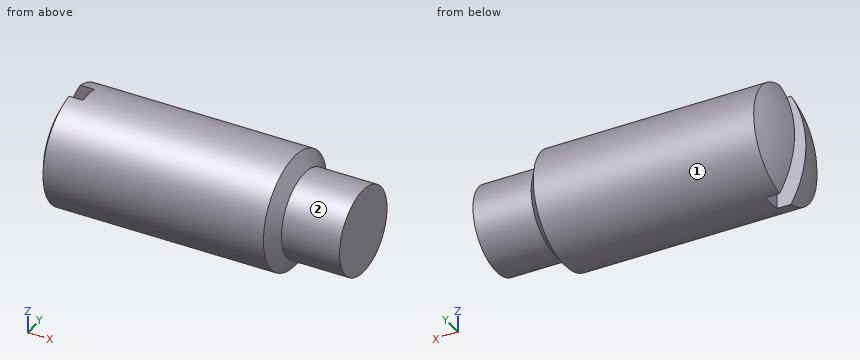
from build123d import *

# Parameters (mm, degrees)
SKETCH2_W  = 19.05
SKETCH2_H  = 3.4036
SLOT_DEPTH = 4.9022


with BuildPart() as part:
    # BodySke → BaseBody (revolve)
    with BuildSketch(Plane.XY, mode=Mode.PRIVATE) as basebody_sk:
        with BuildLine():
            Line((41.0718, 7.1374), (50.8, 7.1374))
            Line((50.8, 7.1374), (50.8, 0))
            Line((50.8, 0), (0, 0))
            ThreePointArc((0, 0), (0.649113009, 4.930502809), (2.552216058, 9.525))
            Line((2.552216058, 9.525), (39.399984482, 9.525))
            Line((39.399984482, 9.525), (41.0718, 7.1374))
        make_face()
    revolve(basebody_sk.sketch.rotate(Axis((-12.7, 0, 0), (1, 0, 0)), 90), axis=Axis((-12.7, 0, 0), (1, 0, 0)))

    # Sketch2 → Slot (cut)
    with BuildSketch(Plane(origin=(0, 0, 0), x_dir=(0, 0, -1), z_dir=(1, 0, 0))):
        Rectangle(SKETCH2_W, SKETCH2_H)
    extrude(amount=SLOT_DEPTH, mode=Mode.SUBTRACT)


solid = part.part
Input: part model. Units: mm. Frame: model coordinates. Face numbers are marked on the shaded views. A direction names the side the tool comes from. Give positions to 0.01 mm unless a question says otherwise; leave off trailing zeros. Write each loop counter-clockwise with the first axis right and the second up, starting at its lowest first coordinate (ties: lowest second). Pieces come first, ordered by that corner, then holes.
Q1. Material intervals for probe 1 along Y at (x, z) = (4, -8); probe 2 along Z at (x, y) = (5.5, -0.25); probe 3 along Y at (x, z) = (9, 1.75), sorted ascending.
Q2. Section C-C, the plane x = 4. Output: boundary loops of the cut face in (y, z) (3 decimals).
Q3. Set-up query: the marked faces 1 and 2. Return all of +Z, -Z, +X, -X, +Y, -Y with unobstructed straight access to the full face (end or side cutting, diameter ignored); none if empty.
Q4. First-contact query: P1, Ø1.4, axis at x = 1.5, z = 0, coming from the -Y side; P2, Ø5, axis at x = 13.5, z = 7, coming from the +Y side (3 decimals); P3, Ø6, axis at x = 44.5, z = 0, coming from the +Y side. Flat tips, straight axial feed; report the tip coordinate or a pass-through.
Q5. Section B-B, the plane y = 0. Output: boundary loops of the cut face in (x, z) (3 decimals), plus the area to 3 significant figures.
Q6. Section D-D, the plane x = 13. Output: boundary loops of the cut face in (y, z) (3 decimals).
Q7. Section A-A, the plane z = 0. Output: boundary loops of the cut face in (x, y) (3 decimals).
Filled in:
1. probe 1: y = -5.17 to -1.7, 1.7 to 5.17
1. probe 2: z = -9.52 to 9.52
1. probe 3: y = -9.36 to 9.36
2. outline: (-1.702, -9.372) - (-1.702, 9.372) arc R9.525 ccw to start; (1.702, -9.372) arc R9.525 ccw to (1.702, 9.372) - close
3. face 1: +X, -X
3. face 2: +X
4. P1: stops at y = -8.89
4. P2: stops at y = 8.395
4. P3: stops at y = 7.14
5. outline: (4.902, -9.525) - (39.4, -9.525) - (41.072, -7.137) - (50.8, -7.137) - (50.8, 7.137) - (41.072, 7.137) - (39.4, 9.525) - (4.902, 9.525) - close
5. area: 824 mm2
6. outline: circle Ø19.05 at (0, 0)
7. outline: (0.076, -1.702) arc R19.05 ccw to (2.552, -9.525) - (39.4, -9.525) - (41.072, -7.137) - (50.8, -7.137) - (50.8, 7.137) - (41.072, 7.137) - (39.4, 9.525) - (2.552, 9.525) arc R19.05 ccw to (0.076, 1.702) - (4.902, 1.702) - (4.902, -1.702) - close
